from build123d import *

# Parameters (mm, degrees)
F0_R     = 2.5
F1_DEPTH = 53.856
F3_DEPTH = 2


with BuildPart() as f1:
    # F0 (on Right) → F1 (new body, symmetric)
    with BuildSketch(Plane.YZ):
        Circle(F0_R)
    extrude(amount=F1_DEPTH, both=True)

    # F2 (on face) → F3 (join)
    with BuildSketch(Plane(origin=(-53.856, 0, 0), x_dir=(0, -1, 0), z_dir=(-1, 0, 0))):
        with BuildLine():
            ThreePointArc((-1, 2.291288), (0, 2.5), (1, 2.291288))
            Line((1, 2.291288), (1, 4.5))
            Line((1, 4.5), (-1, 4.5))
            Line((-1, 4.5), (-1, 2.291288))
        make_face()
        with BuildLine():
            Line((-1, -4.5), (1, -4.5))
            Line((1, -4.5), (1, -2.291288))
            ThreePointArc((1, -2.291288), (0, -2.5), (-1, -2.291288))
            Line((-1, -2.291288), (-1, -4.5))
        make_face()
    extrude(amount=-F3_DEPTH)

    # F4: F1 across plane


with BuildPart() as f1_1:
    add(f1.part)
    add(f1.part.mirror(Plane.YZ))


solid = f1_1.part
The model under review builds one solid part; all positions refer to its coordinate system, in mm. A direction names the side the tool comes from. Give positions to 0.01 mm unless a question says otherwise; leave off trailing zeros. Loops run counter-clockwise (first coordinate to the right, second up) from the corner with the lowest first, then second, coordinate; pieces in that order, holes last. Notation, with made-up numbers: (83, -25.5) -> (103, -25.5) arc R18 cw to (103, -1.5) -> close; hole circle Ø6 at (75, 77). An arc over 180 degrees is marked (long way). Answer as a JSON object with one key per item and string values. Group by question number.
Q1. Tool access review of faces 4 (the flat face through (-53, -1, 3)), 5 (the flat face through (-53, -1, -3)), 6 (the flat face through (53, 1, -3)), 7 (the cylindrical face through (0.75, -0.54, -2.44)): name each direction out of +Z, -Z, +X, -X, +Y, -Y from which nothing blocks a thin tool from reaching the whole face with its end or side.
Q2. Insertion check: pin 1 (1 mm diameter, centred on x = -52.5, z = -3, fed in from +Y); pin 2 (1.6 mm diameter, centred on x = 53, z = 4, fed in from -Y); pin 3 (1 mm diameter, centred on y = -2, z = -2.5, fed in from +X); pin 4 (2 mm diameter, centred on x = 24.5, y = 2, fed in from -Z). Each pin has a flat end and moves straight along its axis. Give the tip position at first contact, or say it passes through.
Q3. Take a section at C-C (x = 21.5). Write out the cut boundary in (y, z).
Q4. Take a section at B-B (y = 0). Write out the cut boundary in (x, z), plus the area to 3 significant figures.
Q5. Wall thickness on line 1 along X through (y, z) = (0.05, -3.75); line 2 along Y through (x, z) = (38.5, 0.25); line 3 along Z through (x, y) = (-33.5, 0.3): over which ranges is each line inside the solid? List them lowest first.
Q6. Draft analysis for pull direction X (two halves, no side actions). For faces 1 (the flat face through (51.856, 0, -3)), 2 (the flat face through (53, 1, 3)), 3 (the flat face through (-53.856, 0, 0)), state which applies: pulls with the +X half, pulls with the -X half, needs draft (parallel to the pull), parting line crosses it, or undercut.
Q7. Take a section at A-A (z = 3.5). Write out the cut boundary in (x, y), plus the area to 3 significant figures.
Answer below:
{
 "1": {"face 4": "+Z, +X, -X, -Y", "face 5": "-Z, +X, -X, -Y", "face 6": "-Z, +X, -X, +Y", "face 7": "none"},
 "2": {"pin 1": "stops at y = 1", "pin 2": "stops at y = -1", "pin 3": "passes through", "pin 4": "stops at z = -2.29"},
 "3": {"outline": "circle Ø5 at (0, 0)"},
 "4": {"outline": "(-53.86, -4.5) -> (-51.86, -4.5) -> (-51.86, -2.5) -> (51.86, -2.5) -> (51.86, -4.5) -> (53.86, -4.5) -> (53.86, 4.5) -> (51.86, 4.5) -> (51.86, 2.5) -> (-51.86, 2.5) -> (-51.86, 4.5) -> (-53.86, 4.5) -> close", "area": "555 mm2"},
 "5": {"line 1": "x = -53.86 to -51.86, 51.86 to 53.86", "line 2": "y = -2.49 to 2.49", "line 3": "z = -2.48 to 2.48"},
 "6": {"face 1": "undercut", "face 2": "needs draft", "face 3": "pulls with the -X half"},
 "7": {"outline": "(-53.86, -1) -> (-51.86, -1) -> (-51.86, 1) -> (-53.86, 1) -> close; (51.86, -1) -> (53.86, -1) -> (53.86, 1) -> (51.86, 1) -> close", "area": "8.00 mm2"}
}
